For this review, take the finished solid that the model builds, in its own axes (mm). A direction names the side the tool comes from. Coordinates: 2 decimals unless noted, no trailing zeros. Order: outer loops, then holes, each group sorted by start corner. A loop starts at its lowest first (then second) coordinate and runs counter-clockwise, first axis right, second up. Notation, with made-up numbers: (66, -6.5) - (97, -6.5) arc R9 ccw to (97, 8.5) - close; hole circle Ø4 at (5, 12). An arc over 180 degrees is marked (long way). One line per item, written item: value. Start each with the question number.
(1) Consider section B-B on x = 6. Write out the cut boundary in (y, z), then the cut area to 3 significant figures.
(2) For faces 5 (the cylindrical face through (-3.905, -19.16, -0.867)), 6 (the flat face through (72.5, 0, 0)), 7 (the cylindrical face through (71.232, 38.536, 0.325)), list the 3-axis set-ups (+Z, -Z, +X, -X, +Y, -Y) from which the entire face can be reached by the end or side of a thin tool; tool diameter is ignored.
(3) Mouldability with a two-part tool opening along Y and no side actions: class faces 1 (the flat face through (0, -80, 0)), 2 (the cylindrical face through (34.51, 3.966, 0.521)), 3 (the flat face through (-2, 40, 0)), 4 (the flat face through (0, 42, 0)) as released by +Y, released by -Y, zero draft, split by the parting line, or undercut.
(4) Consider section A-A on z = 0. Write out the cut boundary in (x, y), then the cut area to 3 significant figures.
(5) To check wall thickness, follow line 1 along X through (y, z) = (-15, -0.25); line 2 along Y through (x, z) = (4, -2.5); line 3 along Y through (x, z) = (63.5, -0.5). State the ranges of each line that lie inside material, in increasing order.
(6) Consider section C-C on y = -32.5. Write out the cut boundary in (x, z).
(7) Clearance check with flat-ended pins moving along their axes: pin 1 (4 mm diameter, centred on x = 40, z = 3, fed in from +Y); pin 2 (2 mm diameter, centred on y = 41.5, z = -1, fed in from -X); pin 3 (1 mm diameter, centred on y = -7.5, z = -1, fed in from -X). State where each tip first meets the part, or that it passes through.
```python
from build123d import *

# Parameters (mm, degrees)
SKETCH1_R           = 4
BOSS_EXTRUDE1_DEPTH = 80
SKETCH3_R           = 4
BOSS_EXTRUDE3_DEPTH = 70
BOSS_EXTRUDE4_START = 40
SKETCH4_R           = 4
BOSS_EXTRUDE4_DEPTH = 40
SKETCH5_R           = 4
BOSS_EXTRUDE5_DEPTH = 70
SKETCH7_R           = 1.5
BOSS_EXTRUDE6_DEPTH = 2.5


with BuildPart() as part:
    # Sketch1 → Boss-Extrude1 (new body)
    with BuildSketch(Plane(origin=(0, 0, 0), x_dir=(1, 0, 0), z_dir=(0, 1, 0))):
        with Locations(Location((0, 0, 0), (0, 0, 270))):
            Circle(SKETCH1_R)
    extrude(amount=-BOSS_EXTRUDE1_DEPTH)

    # Sketch3 → Boss-Extrude3 (add)
    with BuildSketch(Plane(origin=(0, 0, 0), x_dir=(0, 0, -1), z_dir=(1, 0, 0))):
        Circle(SKETCH3_R)
    extrude(amount=BOSS_EXTRUDE3_DEPTH)

    # Sketch4 → Boss-Extrude4 (add)
    with BuildSketch(Plane(origin=(0, 0, 0), x_dir=(1, 0, 0), z_dir=(0, 1, 0)).offset(BOSS_EXTRUDE4_START)):
        with Locations(Location((0, 0, 0), (0, 0, 270))):
            Circle(SKETCH4_R)
    extrude(amount=-BOSS_EXTRUDE4_DEPTH)

    # Sketch5 → Boss-Extrude5 (add)
    with BuildSketch(Plane(origin=(0, 0, 0), x_dir=(0, 0, -1), z_dir=(1, 0, 0))):
        with Locations((0, 40)):
            Circle(SKETCH5_R)
    extrude(amount=BOSS_EXTRUDE5_DEPTH)

    # Sketch7 → Boss-Extrude6 (add)
    with BuildSketch(Plane(origin=(70, 0, 0), x_dir=(0, 0, -1), z_dir=(1, 0, 0))):
        with Locations((0, 40)):
            Circle(SKETCH7_R)
        Circle(SKETCH7_R)
    extrude(amount=BOSS_EXTRUDE6_DEPTH)


solid = part.part
```
Geometry check:
1. outline: circle Ø8 at (0, 0); circle Ø8 at (40, 0)
1. area: 101 mm^2
2. face 5: none
2. face 6: +Z, -Z, +X, +Y, -Y
2. face 7: +X
3. face 1: released by -Y
3. face 2: undercut
3. face 3: released by +Y
3. face 4: zero draft
4. outline: (-4, -80) - (4, -80) - (4, -4) - (70, -4) - (70, -1.5) - (72.5, -1.5) - (72.5, 1.5) - (70, 1.5) - (70, 4) - (4, 4) - (4, 36) - (70, 36) - (70, 38.5) - (72.5, 38.5) - (72.5, 41.5) - (70, 41.5) - (70, 44) - (0, 44) - (0, 40) - (-4, 40) - close
4. area: 2,050 mm^2
5. line 1: x = -3.99 to 3.99
5. line 2: y = -3.12 to 3.12, 36.88 to 43.12
5. line 3: y = -3.97 to 3.97, 36.03 to 43.97
6. outline: circle Ø8 at (0, 0)
7. pin 1: stops at y = 43.87
7. pin 2: stops at x = 0
7. pin 3: stops at x = -3.97
